Could you check a few things on this model? Use its own coordinates, in mm. Face numbers are marked on the shaded views. A direction names the side the tool comes from. Coordinates: 2 decimals unless noted, no trailing zeros. Loops run counter-clockwise (first coordinate to the right, second up) from the corner with the lowest first, then second, coordinate; pieces in that order, holes last. Notation, with made-up numbers: (8.25, 10.25) -> (63.25, 10.25) arc R26 cw to (63.25, 38.25) -> close; hole circle Ø10 at (50, 39.5). An arc over 180 degrees is marked (long way). One line per question, with ' | ' between items.
from build123d import *

# Parameters (mm, degrees)
IZIM1_W                     = 100
IZIM1_H                     = 114
Y_KSEKLIK_EKSTR_ZYON1_DEPTH = 10
IZIM2_W                     = 29.5
IZIM2_H                     = 9.95
KES_EKSTR_ZYON1_DEPTH       = 152.973681932
IZIM3_W                     = 29.5
IZIM3_H                     = 9.95
KES_EKSTR_ZYON2_DEPTH       = 152.973681932
RADYUS1_R                   = 5
KES_EKSTR_ZYON3_DEPTH       = 8


with BuildPart() as part:
    # Çizim1 → Yükseklik-Ekstrüzyon1 (new body)
    with BuildSketch(Plane.XY.offset(10)):
        with Locations((50, 57)):
            Rectangle(IZIM1_W, IZIM1_H)
    extrude(amount=-Y_KSEKLIK_EKSTR_ZYON1_DEPTH)

    # Çizim2 → Kes-Ekstrüzyon1 (cut, through all)
    with BuildSketch(Plane.XY.offset(10)):
        with Locations((50, 101.025)):
            Rectangle(IZIM2_W, IZIM2_H)
    extrude(amount=-KES_EKSTR_ZYON1_DEPTH, mode=Mode.SUBTRACT)

    # Çizim3 → Kes-Ekstrüzyon2 (cut, through all)
    with BuildSketch(Plane(origin=(0, 0, 0), x_dir=(-1, 0, 0), z_dir=(0, 0, -1))):
        with Locations((-50, 12.975)):
            Rectangle(IZIM3_W, IZIM3_H)
    extrude(amount=-KES_EKSTR_ZYON2_DEPTH, mode=Mode.SUBTRACT)

    # Radyus1
    radyus1_edges = [part.edges().sort_by_distance(p)[0] for p in [
        (0, 114, 5),
        (100, 114, 5),
        (100, 0, 5),
        (0, 0, 5),
    ]]
    fillet(radyus1_edges, radius=RADYUS1_R)

    # Çizim14 → Kes-Ekstrüzyon3 (cut)
    with BuildSketch(Plane.XY.offset(10)):
        with BuildLine():
            Line((54.4, 59), (54.4, 55))
            Line((54.4, 55), (56.079473661, 55))
            ThreePointArc((56.079473661, 55), (43.6, 57), (56.079473661, 59))
            Line((56.079473661, 59), (54.4, 59))
        make_face()
    extrude(amount=-KES_EKSTR_ZYON3_DEPTH, mode=Mode.SUBTRACT)


solid = part.part
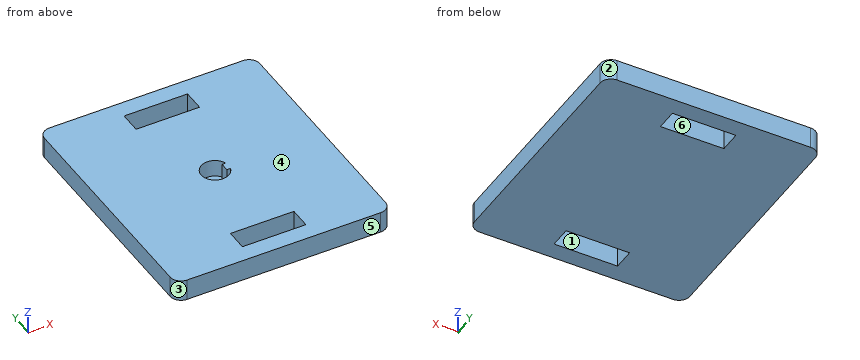
1) I'm going to push a flat-ended pin straight in: pin 1 Ø7.5 at (x, y) = (50, 57) entering from +Z. Where does the tip first touch, or does it pass through?
Data:
pin 1: z = 2
2) If we section it at B-B on z = 8.5: Please give me the cut outline in (x, y).
Data:
outline: (0, 5) arc R5 ccw to (5, 0) -> (95, 0) arc R5 ccw to (100, 5) -> (100, 109) arc R5 ccw to (95, 114) -> (5, 114) arc R5 ccw to (0, 109) -> close; hole (35.25, 8) -> (64.75, 8) -> (64.75, 17.95) -> (35.25, 17.95) -> close; hole (35.25, 96.05) -> (64.75, 96.05) -> (64.75, 106) -> (35.25, 106) -> close; hole (54.4, 55) -> (54.4, 59) -> (56.08, 59) arc R6.4 ccw (long way) to (56.08, 55) -> close
3) If we section it at C-C on y = 57: Please give me the cut outline in (x, z).
Data:
outline: (0, 0) -> (100, 0) -> (100, 10) -> (54.4, 10) -> (54.4, 2) -> (43.6, 2) -> (43.6, 10) -> (0, 10) -> close
4) On a 3-axis mill with a long thin cutter (end or side, diameter ignored), from which of +Z, -Z, +X, -X, +Y, -Y can I reach the whole of each face in a straight line? I mean the marked faces 5 and 6. Say none if no direction works.
Data:
face 5: +Z, -Z, +X, -X, -Y | face 6: +Z, -Z
5) We'd pull the mould along X, two halves only. Please class the marked faces 1, 2, 3 and 4: pulls with the +X half, pulls with the -X half, needs draft (parallel to the pull), parting line crosses it, or undercut.
Data:
face 1: undercut | face 2: pulls with the +X half | face 3: pulls with the -X half | face 4: needs draft
6) I need wall thicknesses on line 1 along Y through (x, z) = (59, 2); line 2 along Y through (x, z) = (50, 7); line 3 along X through (y, z) = (57, 8). Which ranges of each line are inside material? Lowest first, please. Write a range as from..to.
Data:
line 1: 0..8, 17.95..96.05, 106..114 | line 2: 0..8, 17.95..50.6, 63.4..96.05, 106..114 | line 3: 0..43.6, 54.4..100
7) If we section it at A-A on x = 42: Please give me the cut outline in (y, z).
Data:
outline: (0, 0) -> (8, 0) -> (8, 10) -> (0, 10) -> close; (17.95, 0) -> (96.05, 0) -> (96.05, 10) -> (17.95, 10) -> close; (106, 0) -> (114, 0) -> (114, 10) -> (106, 10) -> close
